from build123d import *

# Parameters (mm, degrees)
SKETCH_1_W         = 20
SKETCH_1_H         = 10
BASEPLATE_DEPTH    = 1
EDGEFLANGE_DEPTH   = 20
EDGEFLANGE_2_DEPTH = 20


# Read off the part's stored shape, not the designer's step: EdgeFlange
# Sheet-metal steps are written as plain solids
with BuildPart() as part:
    # Sketch 1 → BasePlate (new body)
    with BuildSketch(Plane.XY):
        with Locations((10, 5)):
            Rectangle(SKETCH_1_W, SKETCH_1_H)
    extrude(amount=-BASEPLATE_DEPTH)

    # EdgeFlange outline → EdgeFlange (cut)
    with BuildSketch(Plane.YZ):
        with BuildLine():
            Line((10, 0), (7.617265824, 0))
            ThreePointArc((7.617265824, 0), (6.605942718, -0.738612788), (5.381197846, -1))
            Line((5.381197846, -1), (10, -1))
            Line((10, -1), (10, 0))
        make_face()
    extrude(amount=EDGEFLANGE_DEPTH, mode=Mode.SUBTRACT)

    # EdgeFlange 2 outline → EdgeFlange 2 (add)
    with BuildSketch(Plane.YZ):
        with BuildLine():
            ThreePointArc((7.617265824, 0), (8.365278527, 1.691353778), (7.979274058, 3.5))
            Line((7.979274058, 3.5), (4.711324865, 9.160254038))
            Line((4.711324865, 9.160254038), (3.845299462, 8.660254038))
            Line((3.845299462, 8.660254038), (7.113248654, 3))
            ThreePointArc((7.113248654, 3), (7.113248654, 1), (5.381197846, 0))
            Line((5.381197846, 0), (7.617265824, 0))
        make_face()
    extrude(amount=EDGEFLANGE_2_DEPTH)


solid = part.part
The model under review builds one solid part; all positions refer to its coordinate system, in mm. A direction names the side the tool comes from. Coordinates: 2 decimals unless noted, no trailing zeros. Loops run counter-clockwise (first coordinate to the right, second up) from the corner with the lowest first, then second, coordinate; pieces in that order, holes last. Notation, with made-up numbers: M -1.75,-21 L 12.25,-21 A21 cw 12.25,5 Z; hole C 32.25,24 d2. An arc over 180 degrees is marked long. Put each result on its own line as item: value. Start each with the question number.
Q1. Wall thickness on line 1 (Z direction, x = 4.5, y = 1.75); line 2 (Z direction, x = 5.75, y = 5.25); line 3 (Z direction, x = 9, y = 4.5): over which ranges is each line inside the solid? List them lowest first.
Q2. The part is to be moulded in two halves that separate along Z. For faces 3 (the flat face through (10, 3, 0)), 4 (the flat face through (20, 7, 4)), 5 (the flat face through (9.86, 6.37, 6.29)), say which applies: +Z half, -Z half, draft (parallel to the pull), parting line (faces both ways), or undercut.
Q3. For faces 1 (the flat face through (9.86, 5.456, 5.87)), 2 (the flat face through (0, 7, 4)), list the 3-axis set-ups (+Z, -Z, +X, -X, +Y, -Y) from which the entire face can be reached by the end or side of a thin tool; tool diameter is ignored.
Q4. Add section A-A (y = 4.5). Write out the cut boundary in (x, z).
Q5. Clearance check with flat-ended pins moving along their axes: pin 1 (5 mm diameter, centred on x = 6, y = 7, fed in from +Z); pin 2 (6 mm diameter, centred on x = 10, z = 7, fed in from +Y); pin 3 (1 mm diameter, centred on y = 6.5, z = 7.5, fed in from +X); pin 4 (2.5 mm diameter, centred on x = 7.5, y = 1.5, fed in from +Z). State where each tip first meets the part, or that it passes through.
Q6. Add section C-C (z = 2). Write out the cut boundary in (x, y).
Q7. Add section D-D (y = 6.5). Write out the cut boundary in (x, z), and give its area (3 significant figures).
Q8. Add section B-B (x = 13.5). Write out the cut boundary in (y, z).
Answers:
1. line 1: z = -1 to 0
1. line 2: z = -1 to 0, 6.23 to 8.23
1. line 3: z = -1 to 0, 7.53 to 9.04
2. face 3: undercut
2. face 4: draft
2. face 5: +Z half
3. face 1: +X, -X, -Y
3. face 2: +Z, -Z, -X, +Y, -Y
4. outline: M 0,-1 L 20,-1 L 20,0 L 0,0 Z; M 0,7.53 L 20,7.53 L 20,9.04 L 0,9.04 Z
5. pin 1: stops at z = 9.16
5. pin 2: stops at y = 7.69
5. pin 3: passes through
5. pin 4: stops at z = 0
6. outline: M 0,7.38 L 20,7.38 L 20,8.38 L 0,8.38 Z
7. outline: M 0,-0.78 L 20,-0.78 L 20,0.34 L 0,0.34 Z; M 0,4.06 L 20,4.06 L 20,6.06 L 0,6.06 Z
7. area: 62.5 mm^2
8. outline: M 0,-1 L 5.38,-1 A3 ccw 7.98,3.5 L 4.71,9.16 L 3.85,8.66 L 7.11,3 A2 cw 5.38,0 L 0,0 Z
